Here's the drawing with two shaded views (mm, measured from the low corner). I have some questions. Coordinates: 2 decimals unless noted, no trailing zeros. Write each loop counter-clockwise with the first axis right and the second up, starting at its lowest first coordinate (ties: lowest second). Pieces come first, ordered by that corner, then holes.
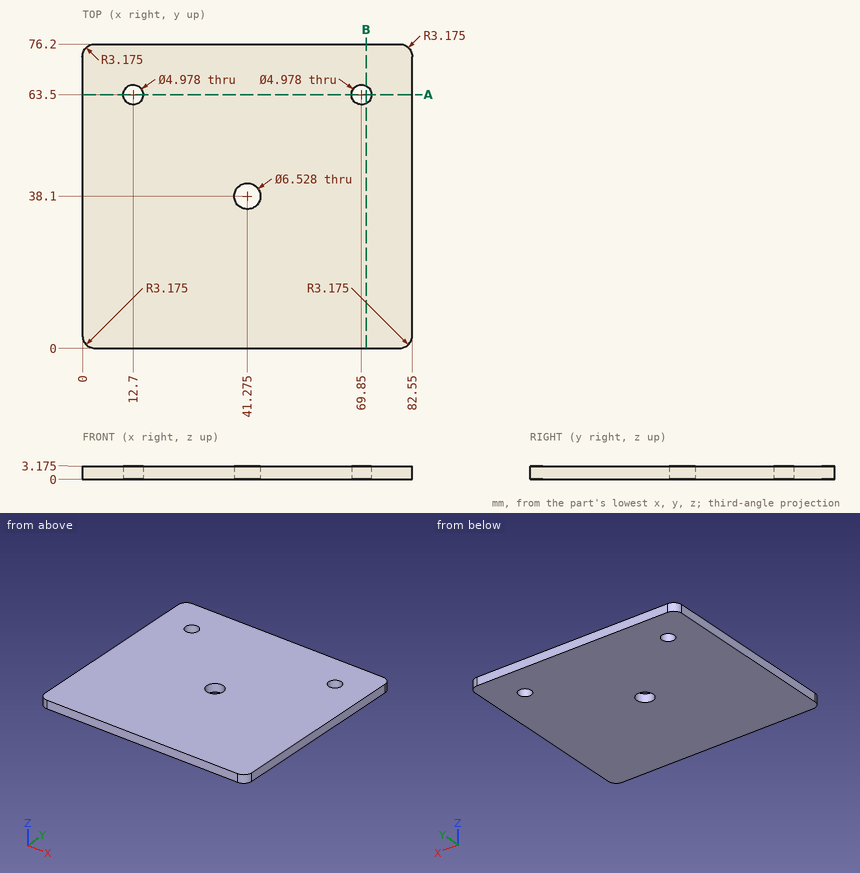
1. I want a section at A-A on y = 63.5. Give the number of separate pieces and of enclosed holes in the cut face.
Verdict:
separate pieces: 3
enclosed holes: 0
2. Please list where these lines run through material, in increasing order: line 1 along Y through (x, z) = (69.85, 1.1); line 2 along X through (y, z) = (38, 2.05); line 3 along Y through (x, z) = (41, 2.8).
Verdict:
line 1: y = 0 to 61.01, 65.99 to 76.2
line 2: x = 0 to 38.01, 44.54 to 82.55
line 3: y = 0 to 34.85, 41.35 to 76.2
3. I want a section at B-B on x = 71. Please give me the cut outline in (y, z) (1 decimal).
Verdict:
outline: (0, 0) - (61.3, 0) - (61.3, 3.2) - (0, 3.2) - close; (65.7, 0) - (76.2, 0) - (76.2, 3.2) - (65.7, 3.2) - close
